Could you check a few things on this model? Use its own coordinates, in mm. Give positions to 0.01 mm unless a question says otherwise; leave off trailing zeros. Write each loop counter-clockwise with the first axis right and the second up, starting at its lowest first coordinate (ties: lowest second). Pieces come first, ordered by that corner, then holes. Notation, with made-up numbers: (10.25, 55.25) - (33.25, 55.25) arc R34 cw to (33.25, 89.25) - close; hole circle Ø11 at (-15, -17). An arc over 180 degrees is marked (long way). Answer in a Markdown table with one row per item.
from build123d import *

# Parameters (mm, degrees)
BOSS_EXTRUDE1_DEPTH = 50
SKETCH2_R           = 2.85
CUT_EXTRUDE1_DEPTH  = 8


with BuildPart() as part:
    # Sketch1 → Boss-Extrude1 (new body)
    with BuildSketch(Plane.XY):
        with BuildLine():
            Line((-9, -3.2), (9, -3.2))
            ThreePointArc((9, -3.2), (9.707106781, -2.907106781), (10, -2.2))
            Line((10, -2.2), (10, 2.2))
            ThreePointArc((10, 2.2), (9.707106781, 2.907106781), (9, 3.2))
            Line((9, 3.2), (-9, 3.2))
            ThreePointArc((-9, 3.2), (-9.707106781, 2.907106781), (-10, 2.2))
            Line((-10, 2.2), (-10, -2.2))
            ThreePointArc((-10, -2.2), (-9.707106781, -2.907106781), (-9, -3.2))
        make_face()
    extrude(amount=BOSS_EXTRUDE1_DEPTH)

    # Sketch2 → Cut-Extrude1 (cut)
    with BuildSketch(Plane(origin=(0, -4, 0), x_dir=(1, 0, 0), z_dir=(0, 1, 0))):
        with Locations(Location((0, -10, 0), (0, 0, 90))):
            Circle(SKETCH2_R)
    extrude(amount=CUT_EXTRUDE1_DEPTH, mode=Mode.SUBTRACT)


solid = part.part
1) We'd pull the mould along X, two halves only. Please class faces 1 (the face through (-0.125, -0.045, 12.847)), 2 (the face through (-10, 0, 25)), 3 (the face through (0, -3.2, 25)), 4 (the face through (9.715, 2.899, 24.65)): +X half, -X half, draft (parallel to the pull), parting line (faces both ways), or undercut.
Check values:
| item | result |
|---|---|
| face 1 | undercut |
| face 2 | -X half |
| face 3 | draft |
| face 4 | +X half |
2) Imagine slicing it at B-B (z = 10). List the corners of the cut face in (x, y) for me, then the cut area to 3 significant figures.
Check values:
| item | result |
|---|---|
| outline | (-10, -2.2) arc R1 ccw to (-9, -3.2) - (-2.85, -3.2) - (-2.85, 3.2) - (-9, 3.2) arc R1 ccw to (-10, 2.2) - close; (2.85, -3.2) - (9, -3.2) arc R1 ccw to (10, -2.2) - (10, 2.2) arc R1 ccw to (9, 3.2) - (2.85, 3.2) - close |
| area | 90.7 mm2 |
3) Imagine slicing it at A-A (x = 0). List the corners of the cut face in (y, z) for me, then the cut area to 3 significant figures.
Check values:
| item | result |
|---|---|
| outline | (-3.2, 0) - (3.2, 0) - (3.2, 7.15) - (-3.2, 7.15) - close; (-3.2, 12.85) - (3.2, 12.85) - (3.2, 50) - (-3.2, 50) - close |
| area | 284 mm2 |
4) If I drill on line 1 (X direction, y = -0.75, z = 10); line 2 (Z direction, x = -0.25, y = -2); line 3 (Z direction, x = -2.25, y = 1.5), over which ranges is the centre line in solid material (lowest first)?
Check values:
| item | result |
|---|---|
| line 1 | x = -10 to -2.85, 2.85 to 10 |
| line 2 | z = 0 to 7.16, 12.84 to 50 |
| line 3 | z = 0 to 8.25, 11.75 to 50 |
5) Imagine slicing it at C-C (y = 0.5). List the corners of the cut face in (x, z) for me, then the cut area to 3 significant figures.
Check values:
| item | result |
|---|---|
| outline | (-10, 0) - (10, 0) - (10, 50) - (-10, 50) - close; hole circle Ø5.7 at (0, 10) |
| area | 974 mm2 |
